from build123d import *

# Parameters (mm, degrees)
IZIM1_R                     = 50
Y_KSEKLIK_EKSTR_ZYON1_DEPTH = 60
BO_ALTMA8_T                 = -5
IZIM2_R                     = 6
KES_EKSTR_ZYON1_DEPTH       = 60
DAIRESEL_KAPLAMA3_COUNT     = 6
IZIM6_R                     = 1.6
KES_EKSTR_ZYON2_DEPTH       = 4
DAIRESEL_KAPLAMA4_COUNT     = 6
IZIM7_W                     = 78
IZIM7_H                     = 120
Y_KSEKLIK_EKSTR_ZYON2_DEPTH = 60
KES_EKSTR_ZYON3_START       = -60
KES_EKSTR_ZYON3_DEPTH       = 60
BO_ALTMA9_T                 = -5
IZIM9_R                     = 6
KES_EKSTR_ZYON4_DEPTH       = 60
DAIRESEL_KAPLAMA5_COUNT     = 6


# Read off the part's stored shape, not the designer's step: M3x0.5 Dişli Delik1
with BuildPart() as part:
    # Çizim1 → Yükseklik-Ekstrüzyon1 (new body)
    with BuildSketch(Plane(origin=(0, 0, 0), x_dir=(1, 0, 0), z_dir=(0, 1, 0))):
        with Locations(Location((0, 0, 0), (0, 0, 270))):
            Circle(IZIM1_R)
    extrude(amount=Y_KSEKLIK_EKSTR_ZYON1_DEPTH)

    # İç Boşaltma8
    bo_altma8_openings = [part.faces().sort_by_distance(p)[0] for p in [
        (0, 0, 0),
    ]]
    offset(amount=BO_ALTMA8_T, openings=bo_altma8_openings, kind=Kind.INTERSECTION)

    # Çizim2 → Kes-Ekstrüzyon1 (cut)
    with BuildSketch(Plane(origin=(0, 60, 0), x_dir=(1, 0, 0), z_dir=(0, 1, 0))):
        with Locations(Location((0, 7, 0), (0, 0, 270))):
            Circle(IZIM2_R)
    extrude(amount=-KES_EKSTR_ZYON1_DEPTH, mode=Mode.SUBTRACT)

    # M3x0.5 Dişli Delik1 outline → M3x0.5 Dişli Delik1 (revolve, cut)
    with BuildSketch(Plane(origin=(15.5, 0, 0), x_dir=(1, 0, 0), z_dir=(0, 0, 1))):
        Polygon((0, 55), (1.25, 55), (1.25, 59.65), (1.6, 60), (0, 60), align=None)
    m3x0_5_di_li_delik1 = revolve(axis=Axis((15.5, 0, 0), (0, 1, 0)), mode=Mode.SUBTRACT)

    # Dairesel Kaplama3: M3x0.5 Dişli Delik1 ×6 about axis
    dairesel_kaplama3_axis = Axis((0, 0, 0), (0, 1, 0))
    for i in range(1, DAIRESEL_KAPLAMA3_COUNT):
        add(m3x0_5_di_li_delik1.rotate(dairesel_kaplama3_axis, i * 360 / DAIRESEL_KAPLAMA3_COUNT), mode=Mode.SUBTRACT)

    # Çizim6 → Kes-Ekstrüzyon2 (cut)
    with BuildSketch(Plane(origin=(0, 60, 0), x_dir=(1, 0, 0), z_dir=(0, 1, 0))):
        with Locations(Location((15.5, 0, 0), (0, 0, 270))):
            Circle(IZIM6_R)
    kes_ekstr_zyon2 = extrude(amount=-KES_EKSTR_ZYON2_DEPTH, mode=Mode.SUBTRACT)

    # Dairesel Kaplama4: Kes-Ekstrüzyon2 ×6 about axis
    dairesel_kaplama4_axis = Axis((0, 0, 0), (0, 1, 0))
    for i in range(1, DAIRESEL_KAPLAMA4_COUNT):
        add(kes_ekstr_zyon2.rotate(dairesel_kaplama4_axis, i * 360 / DAIRESEL_KAPLAMA4_COUNT), mode=Mode.SUBTRACT)

    # Çizim7 → Yükseklik-Ekstrüzyon2 (add)
    with BuildSketch(Plane(origin=(0, 60, 0), x_dir=(1, 0, 0), z_dir=(0, 1, 0))):
        Rectangle(IZIM7_W, IZIM7_H)
    extrude(amount=-Y_KSEKLIK_EKSTR_ZYON2_DEPTH)

    # Çizim8 → Kes-Ekstrüzyon3 (cut)
    with BuildSketch(Plane(origin=(0, 60, 0), x_dir=(1, 0, 0), z_dir=(0, 1, 0)).offset(KES_EKSTR_ZYON3_START)):
        with BuildLine():
            Line((-39, 31.288975694), (-39, -31.288975694))
            ThreePointArc((-39, -31.288975694), (-50, 0), (-39, 31.288975694))
        make_face()
        with BuildLine():
            Line((39, 31.288975694), (39, -31.288975694))
            ThreePointArc((39, -31.288975694), (50, 0), (39, 31.288975694))
        make_face()
    extrude(amount=KES_EKSTR_ZYON3_DEPTH, mode=Mode.SUBTRACT)

    # İç Boşaltma9
    bo_altma9_openings = [part.faces().sort_by_distance(p)[0] for p in [
        (0, 0, 0),
    ]]
    offset(amount=BO_ALTMA9_T, openings=bo_altma9_openings, kind=Kind.INTERSECTION)

    # Çizim9 → Kes-Ekstrüzyon4 (cut)
    with BuildSketch(Plane(origin=(0, 60, 0), x_dir=(1, 0, 0), z_dir=(0, 1, 0))):
        with Locations(Location((0, 7, 0), (0, 0, 270))):
            Circle(IZIM9_R)
    extrude(amount=-KES_EKSTR_ZYON4_DEPTH, mode=Mode.SUBTRACT)

    # Çizim16 → M3x0.5 Dişli Delik3 (revolve, cut)
    with BuildSketch(Plane(origin=(15.5, 60, 0), x_dir=(0, 0, 1), z_dir=(1, 0, 0))):
        Polygon((0, 0), (0, 9.251075774), (1.25, 8.5), (1.25, 0.275), (1.525, 0), align=None)
    m3x0_5_di_li_delik3 = revolve(axis=Axis((15.5, 66.35, 0), (0, -1, 0)), mode=Mode.SUBTRACT)

    # Dairesel Kaplama5: M3x0.5 Dişli Delik3 ×6 about axis
    dairesel_kaplama5_axis = Axis((-0.01225655, 0, 0.085683541), (0, 1, 0))
    for i in range(1, DAIRESEL_KAPLAMA5_COUNT):
        add(m3x0_5_di_li_delik3.rotate(dairesel_kaplama5_axis, i * 360 / DAIRESEL_KAPLAMA5_COUNT), mode=Mode.SUBTRACT)


solid = part.part
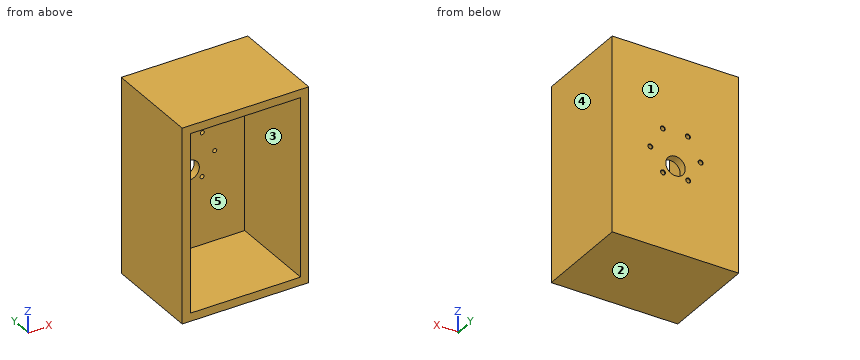
Can you work these out from the model? Positions are in its coordinate system, mm. Face numbers are marked on the shaded views. A direction names the side the tool comes from. Coordinates: 2 decimals unless noted, no trailing zeros. Order: outer loops, then holes, each group sorted by start corner. A loop starts at its lowest first (then second) coordinate and runs counter-clockwise, first axis right, second up. Notation, with made-up numbers: (13, 29.5) - (47, 29.5) arc R25 ccw to (47, 60.5) - close; hole circle Ø5 at (59.25, 52). An arc over 180 degrees is marked (long way). Answer as a JSON object with one key per item and string values. Group by question number.
Q1. On a 3-axis mill with a long thin cutter (end or side, diameter ignored), from which of +Z, -Z, +X, -X, +Y, -Y can I reach the whole of each face in a straight line? I mean the marked faces 4 and 5. Say none if no direction works.
Q2. Imagine slicing it at B-B (y = 17.5). Please give me the cut outline in (x, z), and give its area (3 significant figures).
Q3. I need wall thicknesses on line 1 (Z direction, x = 18.5, y = 53.5); line 2 (X direction, y = 58.3, z = 0); line 3 (X direction, y = 14.5, z = -26.5). Which ranges of each line are inside material? Lowest first, please. Write a range as from..to.
Q4. Imagine slicing it at D-D (x = 28.5). Please give me the cut outline in (y, z), and give its area (3 significant figures).
Q5. Imagine slicing it at C-C (x = 15.5). Please give me the cut outline in (y, z) (3 decimals), and give its area (3 significant figures).
Q6. We'd pull the mould along Z, two halves only. Please class the marked faces 1, 2 and 3: +Z half, -Z half, draft (parallel to the pull), parting line (faces both ways), or undercut.
Q7. Imagine slicing it at A-A (x = 0). Please give me the cut outline in (y, z), and give its area (3 significant figures).
Q8. Will this pin go through, and if not, where does the flat tip stop? P1, Ø3, axis at x = -7.69, z = 13.56, coming from the -Y side.
Determined:
{
 "1": {"face 4": "+Z, -Z, +X, +Y, -Y", "face 5": "-Y"},
 "2": {"outline": "(-39, -60) - (39, -60) - (39, 60) - (-39, 60) - close; hole (-34, -55) - (34, -55) - (34, 55) - (-34, 55) - close", "area": "1,880 mm2"},
 "3": {"line 1": "z = -60..-55, 55..60", "line 2": "x = -39..-16.76, -14.29..14.25, 16.75..39", "line 3": "x = -39..-34, 34..39"},
 "4": {"outline": "(0, -60) - (60, -60) - (60, 60) - (0, 60) - (0, 55) - (55, 55) - (55, -55) - (0, -55) - close", "area": "1,150 mm2"},
 "5": {"outline": "(0, -60) - (60, -60) - (60, -1.525) - (59.725, -1.25) - (55, -1.25) - (55, -55) - (0, -55) - close; (0, 55) - (55, 55) - (55, 1.25) - (59.725, 1.25) - (60, 1.525) - (60, 60) - (0, 60) - close", "area": "1,140 mm2"},
 "6": {"face 1": "draft", "face 2": "-Z half", "face 3": "undercut"},
 "7": {"outline": "(0, -60) - (60, -60) - (60, -13) - (55, -13) - (55, -55) - (0, -55) - close; (0, 55) - (55, 55) - (55, -1) - (60, -1) - (60, 60) - (0, 60) - close", "area": "1,090 mm2"},
 "8": {"P1": "stops at y = 55"}
}
